Autodesk Inventor part; units mm, degrees
ref_plane "YZ Plane" through (0, 0, 0) normal (1, 0, 0) x (0, 1, 0)
ref_plane "XZ Plane" through (0, 0, 0) normal (0, 1, 0) x (-1, 0, 0)
ref_plane "XY Plane" through (0, 0, 0) normal (0, 0, 1) x (1, 0, 0)
sketch "スケッチ1" plane through (0, 0, 0) normal (0, 1, 0) x (-1, 0, 0)
  line L0 (0, 0) -> (17, 0)
  line L1 (17, 0) -> (17, -31.5)
  line L2 (17, -31.5) -> (0, -31.5)
  line L3 (0, -31.5) -> (0, 0)
  dimension "d0" = 17
  dimension "d1" = 31.5
extrude "押し出し1" add sketch "スケッチ1" along normal blind 8
sketch "スケッチ2" plane through (0, 0, 0) normal (1, 0, 0) x (0, 0, -1)
  line L0 (31.5, 0) -> (31.5, 8)
  line L1 (0, 0) -> (31.5, 0)
  point P0 (21.5, 4)
  point P1 (3, 4)
  dimension "d4" = 10
  dimension "d5" = 18.5
  dimension "d6" = 4
  dimension "d7" = 4
hole "穴1" at (0, 4, -21.5) at (0, 4, -3) direction (-1, 0, 0) diameter 2.459 depth 6 tip angle 118
sketch "スケッチ3" plane through (0, 0, -31.5) normal (0, 0, -1) x (-1, 0, 0)
  line L0 (0, 0) -> (17, 0)
  line L1 (0, 0) -> (0, 8)
  point P0 (2.5, 4)
  point P1 (14.5, 4)
  dimension "d15" = 4
  dimension "d16" = 4
  dimension "d17" = 2.5
  dimension "d18" = 12
hole "穴2" at (-2.5, 4, -31.5) at (-14.5, 4, -31.5) direction (0, 0, 1) diameter 2.459 depth 4 tip angle 118
sketch "スケッチ4" plane through (0, 8, 0) normal (0, 1, 0) x (1, 0, 0)
  line L0 (0, 31.5) -> (-17, 31.5)
  line L1 (0, 0) -> (0, 31.5)
  point P0 (-2.5, 26.5)
  point P1 (-14.5, 26.5)
  dimension "d26" = 5
  dimension "d27" = 5
  dimension "d28" = 2.5
  dimension "d29" = 12
hole "穴3" at (-2.5, 8, -26.5) at (-14.5, 8, -26.5) direction (0, -1, 0) diameter 4.1 depth 2.2 tip angle 118
sketch "スケッチ5" plane through (0, 8, 0) normal (0, 1, 0) x (1, 0, 0)
  circle A0 centre (-2.5, 26.5) radius 2.05
  circle A1 centre (-14.5, 26.5) radius 2.05
  point P0 (0, 0)
hole "穴4" at (-2.5, 8, -26.5) at (-14.5, 8, -26.5) at (-2.5, 8, -26.5) at (-14.5, 8, -26.5) direction (0, -1, 0) diameter 2.2 end through all
sketch "スケッチ6" plane through (0, 0, 0) normal (0, -1, 0) x (1, 0, 0)
  circle A0 centre (-14.5, -26.5) radius 2.05
  arc A1 (-2.4721, -27.5996) -> (-2.5279, -27.5996) centre (-2.5, -26.5) ccw
  point P0 (0, 0)
hole "穴5" at (-14.5, 0, -26.5) at (-2.5, 0, -26.5) direction (0, 1, 0) diameter 4.1 depth 2.2 tip angle 118
sketch "スケッチ7" plane through (0, 0, -31.5) normal (0, 0, -1) x (-1, 0, 0)
  line L0 (0, 0) -> (17, 0)
  line L1 (17, 0) -> (17, 8)
  point P0 (8.5, 4)
  dimension "d51" = 4
  dimension "d52" = 8.5
hole "穴6" at (-8.5, 4, -31.5) direction (0, 0, 1) diameter 3 depth 15 tip angle 118
properties part number "本体"
Design review of the part built by this model. Coordinates are the model's own, in mm. A direction names the side the tool comes from. Round coordinates to 2 decimals unless told otherwise and drop trailing zeros. Write each loop counter-clockwise with the first axis right and the second up, starting at its lowest first coordinate (ties: lowest second). Pieces come first, ordered by that corner, then holes. Notation, with made-up numbers: (21.25, 37.5) - (58.25, 37.5) arc R13 ccw to (58.25, 61.5) - close; hole circle Ø9 at (81, 84). An arc over 180 degrees is marked (long way). Use a Markdown table: item, result. Add a question column.
1. We need section A-A (z = -26.5). Count the separate pieces of the cut face and the enclosed holes in it, then the cut area to 3 significant figures.
2. Clearance check with flat-ended pins moving along their axes: pin 1 (1.3 mm diameter, centred on x = -14.5, z = -26.5, fed in from +Y); pin 2 (6.5 mm diameter, centred on x = -14.5, z = -26.5, fed in from +Y); pin 3 (3.5 mm diameter, centred on x = -2.5, z = -26.5, fed in from -Y); pin 4 (2.5 mm diameter, centred on x = -8.5, y = 4, fed in from -Z). State where each tip first meets the part, or that it passes through.
3. For faces 1 (the face through (-15.72, 3.84, -29.47)), 2 (the face through (-2.59, 1.12, -24.45)), 3 (the face through (-3.04, 5.09, -3.57)), 4 (the face through (-2.59, 6.88, -28.55)), list the 3-axis set-ups (+Z, -Z, +X, -X, +Y, -Y) from which the entire face can be reached by the end or side of a thin tool; tool diameter is ignored.
4. We need section B-B (y = 1.25). State the section outline as (x, z) points.
5. Mouldability with a two-part tool opening along Z and no side actions: class faces 5 (the face through (-13.253, 6.885, -28.127)), 6 (the face through (-8, 4, 0)), 7 (the face through (-17, 4, -16)) as +Z half, -Z half, draft (parallel to the pull), parting line (faces both ways), or undercut.
6. Wall thickness on probe 1 along X at (y, z) = (4, -29.5); probe 2 along Z at (x, y) = (-14.5, 0.8); probe 3 along X at (y, z) = (7.55, -26.5): over which ranges is each line inside the solid? List them lowest first.
7. We need section C-C (x = -5.5). State the section outline as (y, z) points.
Output:
| question | item | result |
|---|---|---|
| 1 | separate pieces | 3 |
| 1 | enclosed holes | 1 |
| 1 | area | 74.8 mm2 |
| 2 | pin 1 | passes through |
| 2 | pin 2 | stops at y = 8 |
| 2 | pin 3 | stops at y = 2.38 |
| 2 | pin 4 | stops at z = -16.35 |
| 3 | face 1 | -Z |
| 3 | face 2 | -Y |
| 3 | face 3 | +X |
| 3 | face 4 | +Y |
| 4 | outline | (-17, -31.5) - (0, -31.5) - (0, 0) - (-17, 0) - close; hole circle Ø4.1 at (-14.5, -26.5); hole circle Ø4.1 at (-2.5, -26.5) |
| 5 | face 5 | undercut |
| 5 | face 6 | +Z half |
| 5 | face 7 | draft |
| 6 | probe 1 | x = -17 to -15.73, -13.27 to -10, -7 to -3.73, -1.27 to 0 |
| 6 | probe 2 | z = -31.5 to -28.55, -24.45 to 0 |
| 6 | probe 3 | x = -17 to -16.55, -12.45 to -4.55, -0.45 to 0 |
| 7 | outline | (0, -31.5) - (8, -31.5) - (8, 0) - (0, 0) - close; hole circle Ø2.46 at (4, -21.5); hole circle Ø2.46 at (4, -3) |
